```python
from build123d import *

# Parameters (mm, degrees)
F0_R     = 24.5
F1_DEPTH = 50
F2_R     = 19.75
F3_DEPTH = 4.8
F4_SIZE  = 1


with BuildPart() as f1:
    # F0 (on Top) → F1 (new body)
    with BuildSketch(Plane.XY):
        Circle(F0_R)
    extrude(amount=F1_DEPTH)

    # F2 (on face) → F3 (join)
    with BuildSketch(Plane.XY.offset(50)):
        Circle(F2_R)
    extrude(amount=F3_DEPTH)

    # F4
    f4_edges = [f1.edges().sort_by_distance(p)[0] for p in [
        (-24.5, 0, 0),
        (-19.75, 0, 54.8),
    ]]
    chamfer(f4_edges, length=F4_SIZE)


solid = f1.part
```
The model under review builds one solid part; all positions refer to its coordinate system, in mm. A direction names the side the tool comes from. Round coordinates to 2 decimals unless told otherwise and drop trailing zeros. Order: outer loops, then holes, each group sorted by start corner. A loop starts at its lowest first (then second) coordinate and runs counter-clockwise, first axis right, second up.
(1) For P1, Ø6, axis at x = -13.5, z = 17.5, coming from the -Y side; P2, Ø10, axis at x = -14.5, y = 11, coming from the -Z side; P3, Ø2, axis at y = -15.5, z = 35.5, coming from the +X side; P4, Ø2, axis at y = -16, z = 49, coming from the -X side, all flat-tipped, find the tip position at first contact; note any pin that passes through.
Working result:
P1: stops at y = -22.14
P2: stops at z = 0
P3: stops at x = 19.75
P4: stops at x = -19.37
(2) Tool access review of faces 1 (the face through (2, 20, 50)), 2 (the face through (13.17, 20.66, 25.16)): name each direction out of +Z, -Z, +X, -X, +Y, -Y from which nothing blocks a thin tool from reaching the whole face with its end or side.
Working result:
face 1: +Z
face 2: +Z, -Z
(3) Take a section at C-C, the plane z = 18.5. State the section outline as (x, y) points, plus the area to 3 significant figures.
Working result:
outline: circle Ø49 at (0, 0)
area: 1,890 mm2
(4) Wall thickness on L1, parallel to Z at x = 15, y = -15; L2, parallel to Y at x = -0.5, z = 45; L3, parallel to Y at x = 21, z = 6.5: over which ranges is each line inside the solid? List them lowest first.
Working result:
L1: z = 0 to 50
L2: y = -24.49 to 24.49
L3: y = -12.62 to 12.62
(5) Take a section at A-A, the plane y = 0. State the section outline as (x, z) points.
Working result:
outline: (-24.5, 1) - (-23.5, 0) - (23.5, 0) - (24.5, 1) - (24.5, 50) - (19.75, 50) - (19.75, 53.8) - (18.75, 54.8) - (-18.75, 54.8) - (-19.75, 53.8) - (-19.75, 50) - (-24.5, 50) - close
